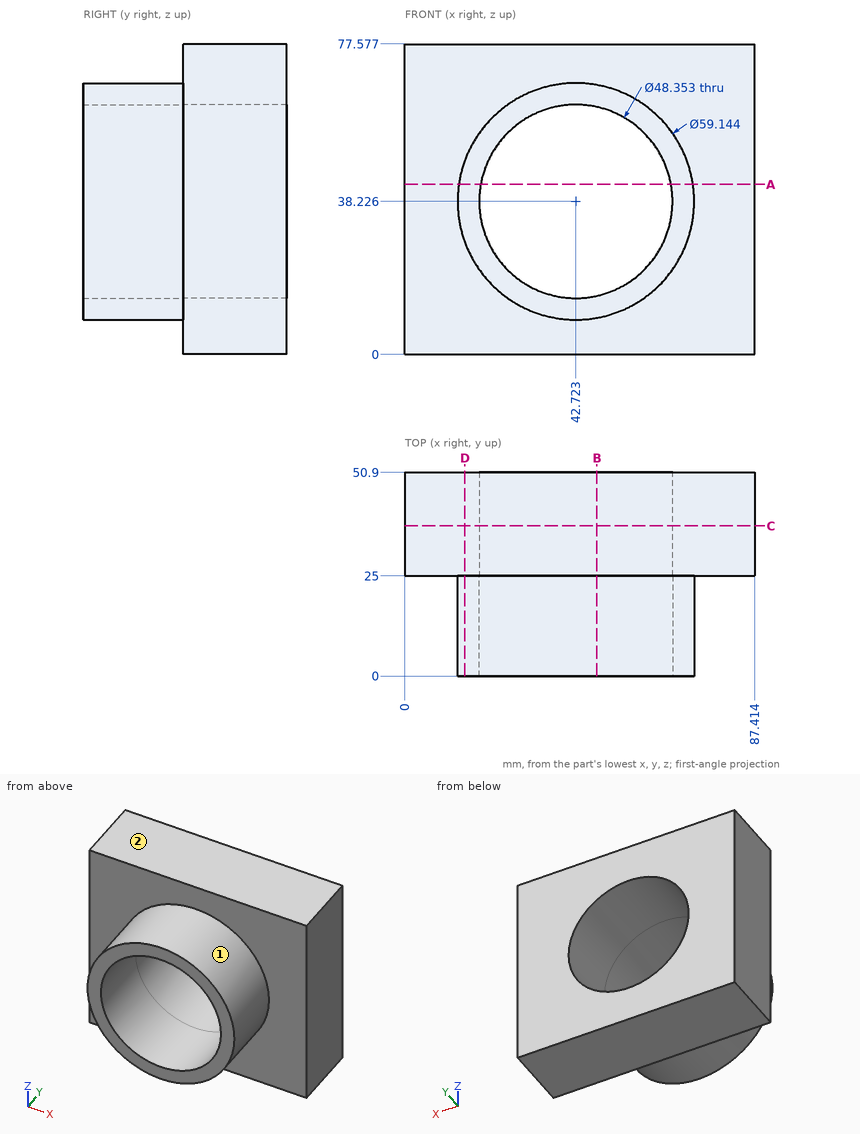
Here's the drawing with two shaded views (mm, measured from the low corner). I have some questions. A direction names the side the tool comes from. Coordinates: 2 decimals unless noted, no trailing zeros. Write each loop counter-clockwise with the first axis right and the second up, starting at its lowest first coordinate (ties: lowest second). Pieces come first, ordered by that corner, then holes. Notation, with made-up numbers: (-20, 49) -> (24, 49) arc R8 ccw to (24, 56) -> close; hole circle Ø1 at (-15.75, 78.25). An arc over 180 degrees is marked (long way). One line per question, with ' | ' between items. Start each with the question number.
1. Please list where these lines run through material, in increasing order: line 1 along X through (y, z) = (47.5, 39) (1 decimal); line 2 along Y through (x, z) = (42.5, 73); line 3 along X through (y, z) = (9.5, 53) (1 decimal).
2. If we section it at C-C (y = 37.5): Please give me the cut outline in (x, z) (1 decimal).
3. If we section it at B-B (x = 48): Please give me the cut outline in (y, z), and give its area (3 significant figures).
4. If we section it at D-D (x = 15): Please give me the cut outline in (y, z) (1 decimal), and give its area (3 significant figures).
5. For the marked faces 1 and 2, which set-ups out of +Z, -Z, +X, -X, +Y, -Y let a thin tool reach every point of the face, with its end or its side?
6. If we section it at A-A (z = 42.5): Please give me the cut outline in (x, y) (1 decimal), and give its area (3 significant figures).
7. Will these pins go through, and if not, where does the flat tip stop? P1, Ø6, axis at y = 20.5, z = 13, coming from the -X side (1 decimal); P2, Ø3, axis at y = 8, z = 63, coming from the -X side; P3, Ø3, axis at x = 70.5, y = 11.5, coming from the -Z side.
Return value:
1) line 1: x = 0 to 18.6, 66.9 to 87.4 | line 2: y = 25 to 50.9 | line 3: x = 17.1 to 23.6, 61.9 to 68.3
2) outline: (0, 0) -> (87.4, 0) -> (87.4, 77.6) -> (0, 77.6) -> close; hole circle Ø48.4 at (42.7, 38.2)
3) outline: (0, 9.13) -> (25, 9.13) -> (25, 0) -> (50.9, 0) -> (50.9, 14.63) -> (0, 14.63) -> close; (0, 61.82) -> (50.9, 61.82) -> (50.9, 77.58) -> (25, 77.58) -> (25, 67.32) -> (0, 67.32) -> close | area: 1,060 mm²
4) outline: (0, 27.9) -> (25, 27.9) -> (25, 0) -> (50.9, 0) -> (50.9, 77.6) -> (25, 77.6) -> (25, 48.5) -> (0, 48.5) -> close | area: 2,520 mm²
5) face 1: -Y | face 2: +Z, +X, -X, +Y, -Y
6) outline: (0, 25) -> (13.5, 25) -> (13.5, 0) -> (18.9, 0) -> (18.9, 50.9) -> (0, 50.9) -> close; (66.5, 0) -> (72, 0) -> (72, 25) -> (87.4, 25) -> (87.4, 50.9) -> (66.5, 50.9) -> close | area: 1,300 mm²
7) P1: stops at x = 23.2 | P2: stops at x = 24.48 | P3: stops at z = 24.66
